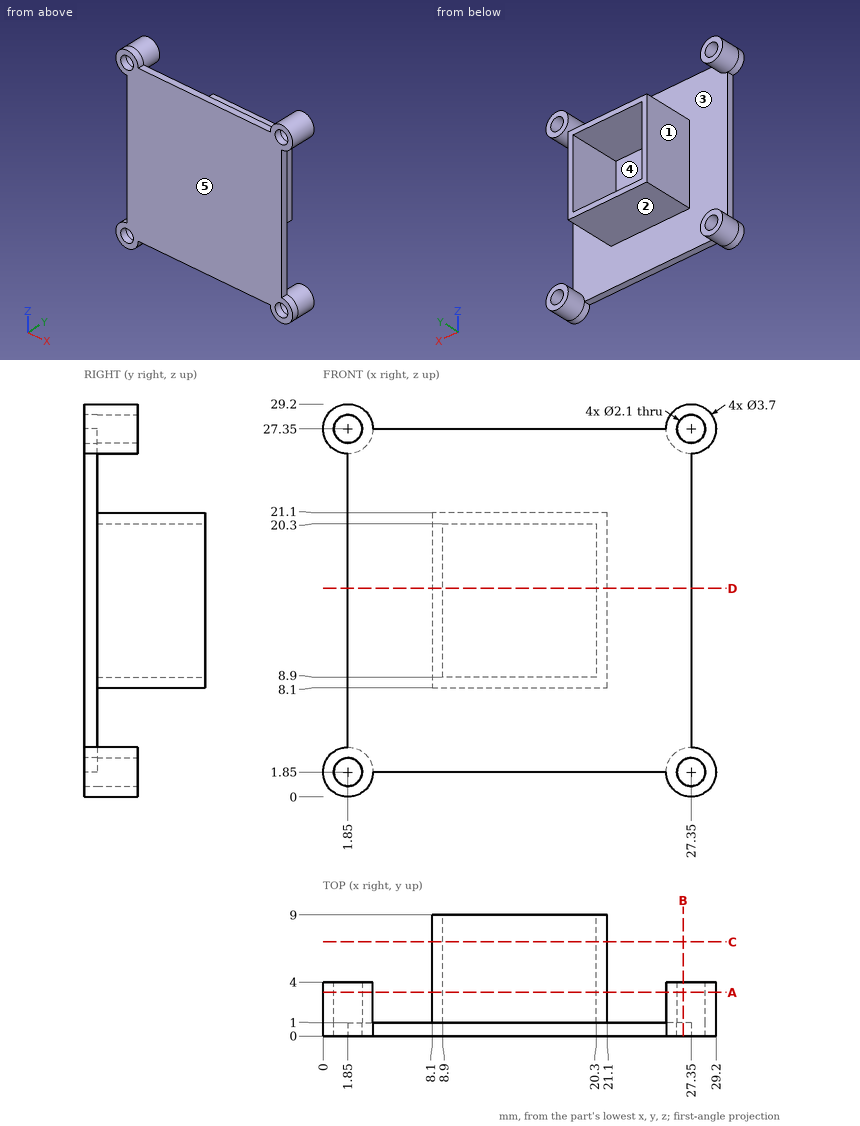
Study the drawing (mm; zero at the part's minimum x, y, z) and answer. A direction names the side the tool comes from. Round coordinates to 2 decimals unless told otherwise and drop trailing zeros. Loops run counter-clockwise (first coordinate to the right, second up) from the corner with the lowest first, then second, coordinate; pieces in that order, holes last.
Q1. Which of the six approach directions +Z, -Z, +X, -X, +Y, -Y give full straight-line access (tool end or side, diameter ignored) to the marked faces 4 and 5?
Q2. Given pin 1 Ø4 at (y, z) = (6, 17.5) entering from +X; pin 2 Ø3.5 at (x, z) = (1.85, 1.85) entering from +Y; pin 3 Ø1.5 at (x, y) = (22, 6) entering from -Z; pin 4 Ø1.5 at (x, y) = (21.5, 1.5) entering from +Z, each flat-ended and moving along its own axis, determine where each tip first touches the part or whether it passes through.
Q3. Section C-C, the plane y = 7 is taken. Determine the outline of the cut face in (x, z), then the cut area to 3 significant figures.
Q4. Section B-B, the plane x = 26.75 is taken. Determine the outline of the cut face in (y, z), then the cut area to 3 significant figures.
Q5. For a pull along X with two mould halves and no side action, classify the marked faces 1, 2 and 3 as released by +X, released by -X, zero draft, split by the parting line, or undercut.
Q6. Find the intervals of material crossed by line 1 (X direction, y = 2.95, z = 27.35); line 2 (X direction, y = 2, z = 1.5); line 3 (Z direction, x = 10.75, y = 1.5), in increasing order.
Q7. Section A-A, the plane y = 3.25 is taken. Count the separate pieces of the cut face and the enclosed holes in it, then the cut area to 3 significant figures.
Q8. Section D-D, the plane z = 15.5 is taken. Determine the outline of the cut face in (x, y), then the cut area to 3 significant figures.
Completed:
1. face 4: +Y
1. face 5: +Z, -Z, +X, -X, -Y
2. pin 1: stops at x = 21.1
2. pin 2: stops at y = 4
2. pin 3: passes through
2. pin 4: stops at z = 27.35
3. outline: (8.1, 8.1) - (21.1, 8.1) - (21.1, 21.1) - (8.1, 21.1) - close; hole (8.9, 8.9) - (20.3, 8.9) - (20.3, 20.3) - (8.9, 20.3) - close
3. area: 39.0 mm2
4. outline: (0, 0.1) - (4, 0.1) - (4, 0.99) - (0, 0.99) - close; (0, 2.71) - (4, 2.71) - (4, 3.6) - (1, 3.6) - (1, 25.6) - (4, 25.6) - (4, 26.49) - (0, 26.49) - close; (0, 28.21) - (4, 28.21) - (4, 29.1) - (0, 29.1) - close
4. area: 36.2 mm2
5. face 1: released by -X
5. face 2: zero draft
5. face 3: undercut
6. line 1: x = 0 to 0.8, 2.9 to 3.7, 25.5 to 26.3, 28.4 to 29.2
6. line 2: x = 0.03 to 0.86, 2.84 to 3.67, 25.53 to 26.36, 28.34 to 29.17
6. line 3: z = 8.1 to 8.9, 20.3 to 21.1
7. separate pieces: 5
7. enclosed holes: 5
7. area: 68.2 mm2
8. outline: (1.85, 0) - (27.35, 0) - (27.35, 1) - (21.1, 1) - (21.1, 9) - (20.3, 9) - (20.3, 1) - (8.9, 1) - (8.9, 9) - (8.1, 9) - (8.1, 1) - (1.85, 1) - close
8. area: 38.3 mm2
